```python
from build123d import *

# Parameters (mm, degrees)
SKETCH_1_W          = 80
SKETCH_1_H          = 180
EXTRUDE_1_DEPTH     = 5
HOLE_WIZARD_2_D     = 4.5
HOLE_WIZARD_3_D     = 23
HOLE_WIZARD_4_D     = 9
SKETCH_12_W         = 80
SKETCH_12_H         = 110
CUT_EXTRUDE_1_DEPTH = 10
SKETCH_13_W         = 80
SKETCH_13_H         = 60
EXTRUDE_2_DEPTH     = 5
SKETCH_14_W         = 30
SKETCH_14_H         = 130
EXTRUDE_3_DEPTH     = 5
SKETCH_15_W         = 140
SKETCH_15_H         = 8
CUT_EXTRUDE_2_DEPTH = 10
SKETCH_16_W         = 140
SKETCH_16_H         = 18
EXTRUDE_4_DEPTH     = 5
HOLE_WIZARD_5_D     = 9
HOLE_WIZARD_5_DEPTH = 2
HOLE_WIZARD_6_D     = 3.5
HOLE_WIZARD_7_D     = 3.5
SKETCH_26_W         = 140
SKETCH_26_H         = 21.5
CUT_EXTRUDE_3_DEPTH = 10
HOLE_WIZARD_8_D     = 3.5
SKETCH_30_W         = 15
SKETCH_30_H         = 15
CUT_EXTRUDE_4_DEPTH = 163.441527942
HOLE_WIZARD_9_D     = 3.5
CUT_EXTRUDE_5_DEPTH = 10
HOLE_WIZARD_10_D    = 3.3


with BuildPart() as part:
    # 草图1 → 凸台-拉伸1 (new body)
    with BuildSketch(Plane(origin=(0, 0, 0), x_dir=(1, 0, 0), z_dir=(0, 1, 0))):
        Rectangle(SKETCH_1_W, SKETCH_1_H)
    extrude(amount=EXTRUDE_1_DEPTH)

    # 孔2 (through all)
    with Locations(Plane(origin=(0, 5, 0), x_dir=(1, 0, 0), z_dir=(0, 1, 0))):
        with Locations((0, -79), (25.11473671, -35.5), (-25.11473671, -35.5)):
            Hole(HOLE_WIZARD_2_D / 2)

    # 孔3 (through all)
    with Locations(Plane(origin=(0, 5, 0), x_dir=(1, 0, 0), z_dir=(0, 1, 0))):
        with Locations((0, -50)):
            Hole(HOLE_WIZARD_3_D / 2)

    # 孔4 (through all)
    with Locations(Plane(origin=(0, 5, 0), x_dir=(1, 0, 0), z_dir=(0, 1, 0))):
        with Locations((0, -69.25)):
            Hole(HOLE_WIZARD_4_D / 2)

    # 草图12 → 切除-拉伸1 (cut)
    with BuildSketch(Plane(origin=(0, 5, 0), x_dir=(1, 0, 0), z_dir=(0, 1, 0))):
        with Locations((0, 35)):
            Rectangle(SKETCH_12_W, SKETCH_12_H)
    extrude(amount=-CUT_EXTRUDE_1_DEPTH, mode=Mode.SUBTRACT)

    # 草图13 → 凸台-拉伸2 (add)
    with BuildSketch(Plane(origin=(0, 5, 0), x_dir=(1, 0, 0), z_dir=(0, 1, 0))):
        with Locations((0, -120)):
            Rectangle(SKETCH_13_W, SKETCH_13_H)
    extrude(amount=-EXTRUDE_2_DEPTH)

    # 草图14 → 凸台-拉伸3 (add)
    with BuildSketch(Plane(origin=(0, 5, 0), x_dir=(1, 0, 0), z_dir=(0, 1, 0))):
        with Locations((-55, -85)):
            Rectangle(SKETCH_14_W, SKETCH_14_H)
        with Locations((55, -85)):
            Rectangle(SKETCH_14_W, SKETCH_14_H)
    extrude(amount=-EXTRUDE_3_DEPTH)

    # 草图15 → 切除-拉伸2 (cut)
    with BuildSketch(Plane(origin=(0, 5, 0), x_dir=(1, 0, 0), z_dir=(0, 1, 0))):
        with Locations((0, -24)):
            Rectangle(SKETCH_15_W, SKETCH_15_H)
    extrude(amount=-CUT_EXTRUDE_2_DEPTH, mode=Mode.SUBTRACT)

    # 草图16 → 凸台-拉伸4 (add)
    with BuildSketch(Plane(origin=(0, 5, 0), x_dir=(1, 0, 0), z_dir=(0, 1, 0))):
        with Locations((0, -159)):
            Rectangle(SKETCH_16_W, SKETCH_16_H)
    extrude(amount=-EXTRUDE_4_DEPTH)

    # 孔5
    with Locations(Plane(origin=(0, 0, 0), x_dir=(-1, 0, 0), z_dir=(0, -1, 0))):
        with Locations((0, -79)):
            Hole(HOLE_WIZARD_5_D / 2, depth=HOLE_WIZARD_5_DEPTH)

    # 孔6 (through all)
    with Locations(Plane(origin=(0, 0, 0), x_dir=(-1, 0, 0), z_dir=(0, -1, 0))):
        with Locations((-49.5, -44.5), (-49.5, -110), (66.5, -110), (66.5, -44.5)):
            Hole(HOLE_WIZARD_6_D / 2)

    # 孔7 (through all)
    with Locations(Plane(origin=(0, 5, 0), x_dir=(1, 0, 0), z_dir=(0, 1, 0))):
        with Locations((-66.5, -117), (-12.5, -117), (-12.5, -143), (-66.5, -143)):
            hole_wizard_7 = Hole(HOLE_WIZARD_7_D / 2)

    # 镜向1: 孔7 across plane
    add(hole_wizard_7.mirror(Plane.ZY), mode=Mode.SUBTRACT)

    # 草图26 → 切除-拉伸3 (cut)
    with BuildSketch(Plane(origin=(0, 5, 0), x_dir=(1, 0, 0), z_dir=(0, 1, 0))):
        with Locations((0, -157.25)):
            Rectangle(SKETCH_26_W, SKETCH_26_H)
    extrude(amount=-CUT_EXTRUDE_3_DEPTH, mode=Mode.SUBTRACT)

    # 孔8 (through all)
    with Locations(Plane(origin=(0, 5, 0), x_dir=(1, 0, 0), z_dir=(0, 1, 0))):
        with Locations((-66.5, -31.5), (66.5, -31.5)):
            Hole(HOLE_WIZARD_8_D / 2)

    # 草图30 → 切除-拉伸4 (cut, through all)
    with BuildSketch(Plane.XZ):
        with Locations((7.5, 130)):
            Rectangle(SKETCH_30_W, SKETCH_30_H)
        with Locations((-7.5, 130)):
            Rectangle(SKETCH_30_W, SKETCH_30_H)
    extrude(amount=-CUT_EXTRUDE_4_DEPTH, mode=Mode.SUBTRACT)

    # 孔9 (through all)
    with Locations(Plane(origin=(0, 0, 0), x_dir=(-1, 0, 0), z_dir=(0, -1, 0))):
        with Locations((-66.5, -65)):
            Hole(HOLE_WIZARD_9_D / 2)

    # 草图37 → 切除-拉伸5 (cut)
    with BuildSketch(Plane(origin=(0, 0, 0), x_dir=(-1, 0, 0), z_dir=(0, -1, 0))):
        Polygon((-67, -76.732050808), (-67, -96.5), (-53, -96.5), (-53, -84.814954576), align=None)
    extrude(amount=-CUT_EXTRUDE_5_DEPTH, mode=Mode.SUBTRACT)

    # 孔10 (through all)
    with Locations(Plane(origin=(0, 0, 0), x_dir=(-1, 0, 0), z_dir=(0, -1, 0))):
        with Locations((-57, -100.75), (-57, -142.25), (31, -142.25)):
            Hole(HOLE_WIZARD_10_D / 2)


solid = part.part
```
Geometry check sheet. Reference: the model listing, model coordinates, mm. A direction names the side the tool comes from. Give positions to 0.01 mm unless a question says otherwise; leave off trailing zeros. Loops run counter-clockwise (first coordinate to the right, second up) from the corner with the lowest first, then second, coordinate; pieces in that order, holes last. Notation, with made-up numbers: (-13.5, 49) - (6.5, 49) arc R30 ccw to (6.5, 76) - close; hole circle Ø6 at (-26, 43). An arc over 180 degrees is marked (long way). Use CSV: the item, a comma, the result in double quotes. Start each with the question number.
Q1. Section check D-D, the plane x = 49.5. Record the cut outline in (y, z).
Q2. Access from +Z, -Z, +X, -X, +Y, -Y to the whole of each face (thin tool, end or side, straight path). Record for faces 4 (the face through (0, 2, 137.5)), 5 (the face through (-1, 3, 146.5)), 6 (the face through (-0.59, 1.01, 74.54)).
Q3. Section check B-B, the plane x = -31. Record the cut outline in (y, z), and give its area (3 significant figures).
Q4. Scan lines: probe 1 along Z at (x, y) = (-66.5, 2.75); probe 2 along Z at (x, y) = (12.5, 2.3); probe 3 along X at (y, z) = (2.25, 31.5). Record each from-to range of solid material in increasing order. Write a range as from..to.
Q5. Section check C-C, the plane z = 117. Record the cut outline in (x, y), and give its area (3 significant figures).
Q6. Release check for a two-part mould opening along X. For faces 1 (the face through (55.69, 2.53, 101.75)), 2 (the face through (2.493, 2.465, 61.227)), 3 (the face through (-1, 0, 86)) record: +X half, -X half, draft (parallel to the pull), parting line (faces both ways), or undercut.
Q7. Section check A-A, the plane z = 100.75. Record the cut outline in (x, y), and give its area (4 significant figures).
Findings below:
1,outline,"(0, 28) - (5, 28) - (5, 42.75) - (0, 42.75) - close; (0, 46.25) - (5, 46.25) - (5, 108.25) - (0, 108.25) - close; (0, 111.75) - (5, 111.75) - (5, 146.5) - (0, 146.5) - close"
2,face 4,"+Y, -Y"
2,face 5,"+Z, +X, -X, +Y, -Y"
2,face 6,"-Y"
3,outline,"(0, 28) - (5, 28) - (5, 140.6) - (0, 140.6) - close; (0, 143.9) - (5, 143.9) - (5, 146.5) - (0, 146.5) - close"
3,area,"576 mm^2"
4,probe 1,"z = 28..29.75, 33.25..42.75, 46.25..108.25, 111.75..115.25, 118.75..141.25, 144.75..146.5"
4,probe 2,"z = 28..115.25, 118.75..122.5, 137.5..141.25, 144.75..146.5"
4,probe 3,"x = -70..-68.25, -64.75..64.75, 68.25..70"
5,outline,"(-70, 0) - (-68.25, 0) - (-68.25, 5) - (-70, 5) - close; (-64.75, 0) - (-14.25, 0) - (-14.25, 5) - (-64.75, 5) - close; (-10.75, 0) - (10.75, 0) - (10.75, 5) - (-10.75, 5) - close; (14.25, 0) - (64.75, 0) - (64.75, 5) - (14.25, 5) - close; (68.25, 0) - (70, 0) - (70, 5) - (68.25, 5) - close"
5,area,"630 mm^2"
6,face 1,"undercut"
6,face 2,"undercut"
6,face 3,"draft"
7,outline,"(-70, 0) - (55.35, 0) - (55.35, 5) - (-70, 5) - close; (58.65, 0) - (70, 0) - (70, 5) - (58.65, 5) - close"
7,area,"683.5 mm^2"
